from build123d import *

# Parameters (mm, degrees)
SKETCH_1_R          = 20
EXTRUDE_1_DEPTH     = 50
SKETCH_2_W          = 30
SKETCH_2_H          = 10
CUT_EXTRUDE_1_DEPTH = 4


with BuildPart() as part:
    # 草图1 → 凸台-拉伸1 (new body)
    with BuildSketch(Plane.XY):
        Circle(SKETCH_1_R)
    extrude(amount=-EXTRUDE_1_DEPTH)

    # 草图2 → 切除-拉伸1 (cut)
    with BuildSketch(Plane(origin=(0, 0, 0), x_dir=(1, 0, 0), z_dir=(0, 1, 0))):
        with Locations((25, 0)):
            Rectangle(SKETCH_2_W, SKETCH_2_H)
    extrude(amount=-CUT_EXTRUDE_1_DEPTH, mode=Mode.SUBTRACT)


solid = part.part
The listing builds one solid part. Answer for the finished solid, in the listing's coordinates (mm). A direction names the side the tool comes from. Give positions to 0.01 mm unless a question says otherwise; leave off trailing zeros. Write each loop counter-clockwise with the first axis right and the second up, starting at its lowest first coordinate (ties: lowest second). Pieces come first, ordered by that corner, then holes. Notation, with made-up numbers: (-19, 31) -> (21, 31) arc R20 ccw to (21, 36) -> close; hole circle Ø7 at (6, 52). An arc over 180 degrees is marked (long way). Use a Markdown table: item, result.
(1) Section A-A, the plane y = 16 is taken. Determine the outline of the cut face in (x, z), then the cut area to 3 significant figures.
Return value:
| item | result |
|---|---|
| outline | (-12, -50) -> (12, -50) -> (12, 0) -> (-12, 0) -> close |
| area | 1,200 mm2 |
(2) Determine the mould class of faces 1 (the flat face through (0, 0, 0)), 2 (the cylindrical face through (-4.336, -19.524, -24.65)), 3 (the flat face through (15, -4, -3)), 4 (the flat face through (15, 0, -3)) for opening direction Y: released by +Y, released by -Y, zero draft, split by the parting line, or undercut.
Return value:
| item | result |
|---|---|
| face 1 | zero draft |
| face 2 | split by the parting line |
| face 3 | undercut |
| face 4 | undercut |
(3) Find the intervals of material crossed by probe 1 along Y at (x, z) = (2, -20); probe 2 along X at (y, z) = (-8, -25); probe 3 along Y at (x, z) = (15, -39), in increasing order. Write a range as from..to.
Return value:
| item | result |
|---|---|
| probe 1 | -19.9..19.9 |
| probe 2 | -18.33..18.33 |
| probe 3 | -13.23..13.23 |
(4) Section C-C, the plane z = -32 is taken. Determine the outline of the cut face in (x, y), then the cut area to 3 significant figures.
Return value:
| item | result |
|---|---|
| outline | circle Ø40 at (0, 0) |
| area | 1,260 mm2 |
(5) Section D-D, the plane y = -12 is taken. Determine the outline of the cut face in (x, z).
Return value:
| item | result |
|---|---|
| outline | (-16, -50) -> (16, -50) -> (16, 0) -> (-16, 0) -> close |
(6) Flat-ended cylindrical pins translate along their axes: P1, Ø2.5, axis at x = 16.5, z = -1.5, coming from the -Y side; P2, Ø6, axis at x = 15.5, z = -13, coming from the -Y side; P3, Ø1.2, axis at x = 15, y = -1, coming from the +Z side. Find the tip coordinate at first contact, or state that the pin passes through.
Return value:
| item | result |
|---|---|
| P1 | y = -12.94 |
| P2 | y = -15.61 |
| P3 | z = -5 |
(7) Section B-B, the plane x = 17.5 is taken. Determine the outline of the cut face in (y, z).
Return value:
| item | result |
|---|---|
| outline | (-9.68, -50) -> (9.68, -50) -> (9.68, 0) -> (0, 0) -> (0, -5) -> (-4, -5) -> (-4, 0) -> (-9.68, 0) -> close |
(8) For faces 5 (the flat face through (0, 0, -50)), 6 (the flat face through (15, -2, -5)), determine the directions among +Z, -Z, +X, -X, +Y, -Y from which every point of the face is accessible in a straight line to the end or side of a thin tool.
Return value:
| item | result |
|---|---|
| face 5 | -Z, +X, -X, +Y, -Y |
| face 6 | +Z, +X |
